Verification items for this drawing (mm, ordinates from the low corner). A direction names the side the tool comes from. Round coordinates to 2 decimals unless told otherwise and drop trailing zeros. Order: outer loops, then holes, each group sorted by start corner. A loop starts at its lowest first (then second) coordinate and runs counter-clockwise, first axis right, second up. Notation, with made-up numbers: (-22.5, -38) - (4.5, -38) arc R26 ccw to (4.5, -3) - close; hole circle Ø8 at (20, 70). An arc over 180 degrees is marked (long way). One line per question, with ' | ' between items. Start each with the question number.
Q1. Sectioned sample at A-A, the plane z = 4. Enter the section's corners in (x, y).
Q2. Material ranges on line 1 along X through (y, z) = (0.6, 12); line 2 along X through (y, z) = (0.35, 16.5); line 3 along Y through (x, z) = (15.5, 2.25), recorded low to high.
Q3. Sectioned sample at C-C, the plane x = 1.75. Enter the section's corners in (y, z).
Q4. Tool access check on the marked faces 1 and 2. Record the directions out of +Z, -Z, +X, -X, +Y, -Y that give a thin tool (end or side, any length) a straight path to the whole face; none if there is none.
Q5. Mould release check, pull along X, two halves, no side actions. Record for the marked faces 3 and 4: +X half, -X half, draft (parallel to the pull), parting line (faces both ways), or undercut.
Q6. Gauge pin test, flat end, axial feed: P1, Ø1.5, axis at x = 18.5, z = 9, coming from the -Y side. Record the tip position at first contact, or that the pin passes through.
Q7. Sectioned sample at B-B, the plane x = 15.75. Enter the section's corners in (y, z).
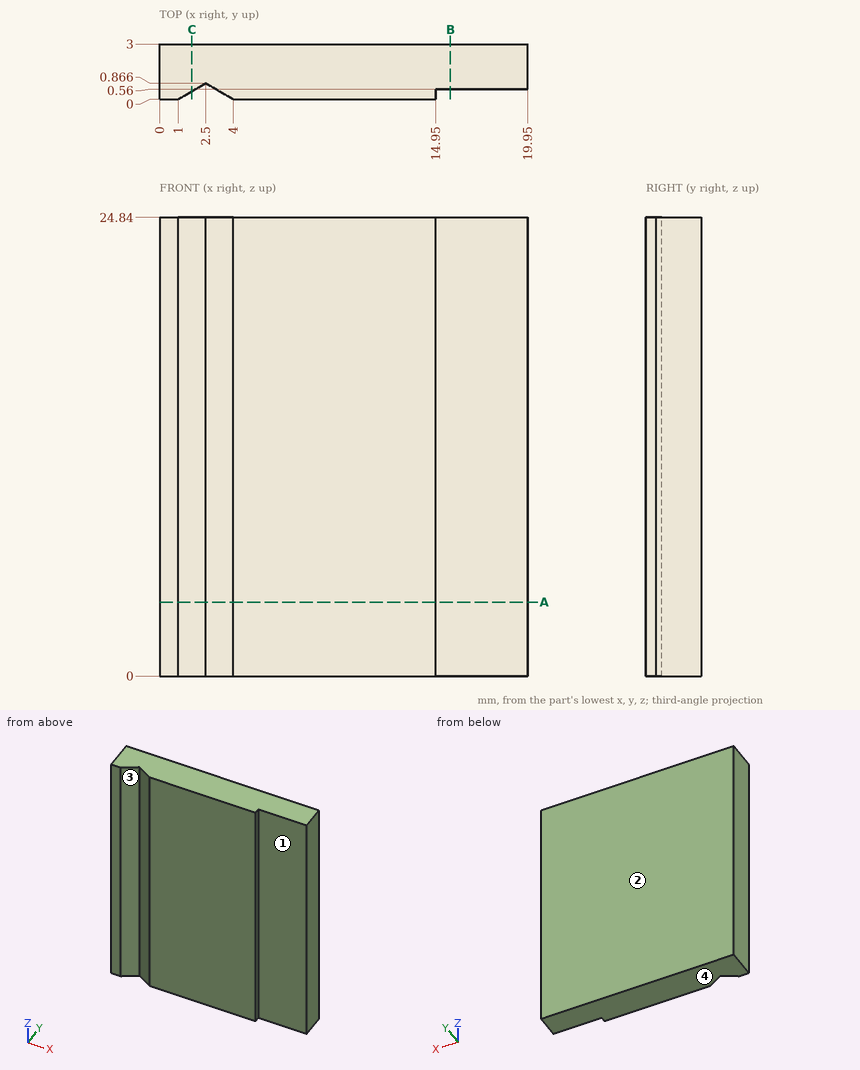
Determined:
1) outline: (0, 0) - (1, 0) - (2.5, 0.87) - (4, 0) - (14.95, 0) - (14.95, 0.56) - (19.95, 0.56) - (19.95, 3) - (0, 3) - close
2) line 1: x = 0 to 2.04, 2.96 to 19.95 | line 2: x = 0 to 1.61, 3.39 to 14.95 | line 3: y = 0.56 to 3
3) outline: (0.43, 0) - (3, 0) - (3, 24.84) - (0.43, 24.84) - close
4) face 1: +Z, -Z, +X, -Y | face 2: +Z, -Z, +X, -X, +Y
5) face 3: undercut | face 4: draft
6) P1: stops at y = 0.56
7) outline: (0.56, 0) - (3, 0) - (3, 24.84) - (0.56, 24.84) - close
